```python
from build123d import *

# Parameters (mm, degrees)
PACK_PLINT_IZGARA_PANELI_1_START  = 18.5
SKETCH1_W                         = 580
SKETCH1_H                         = 80
PACK_PLINT_IZGARA_PANELI_1_DEPTH  = 1.5
PACK_PLINT_IZGARA_PANELI_2_START  = 17
SKETCH2_W                         = 20
SKETCH2_H                         = 60
PACK_PLINT_IZGARA_PANELI_2_DEPTH  = 4
PACK_PLINT_IZGARA_PANELI_3_START  = 17
SKETCH3_W                         = 20
SKETCH3_H                         = 60
PACK_PLINT_IZGARA_PANELI_3_DEPTH  = 4
PACK_PLINT_IZGARA_PANELI_4_START  = 17
SKETCH4_W                         = 20
SKETCH4_H                         = 60
PACK_PLINT_IZGARA_PANELI_4_DEPTH  = 4
PACK_PLINT_IZGARA_PANELI_5_START  = 17
SKETCH5_W                         = 20
SKETCH5_H                         = 60
PACK_PLINT_IZGARA_PANELI_5_DEPTH  = 4
PACK_PLINT_IZGARA_PANELI_6_START  = 17
SKETCH6_W                         = 20
SKETCH6_H                         = 60
PACK_PLINT_IZGARA_PANELI_6_DEPTH  = 4
PACK_PLINT_IZGARA_PANELI_7_START  = 17
SKETCH7_W                         = 20
SKETCH7_H                         = 60
PACK_PLINT_IZGARA_PANELI_7_DEPTH  = 4
PACK_PLINT_IZGARA_PANELI_8_START  = 17
SKETCH8_W                         = 20
SKETCH8_H                         = 60
PACK_PLINT_IZGARA_PANELI_8_DEPTH  = 4
PACK_PLINT_IZGARA_PANELI_9_START  = 17
SKETCH9_W                         = 20
SKETCH9_H                         = 60
PACK_PLINT_IZGARA_PANELI_9_DEPTH  = 4
PACK_PLINT_IZGARA_PANELI_10_START = 17
SKETCH10_W                        = 20
SKETCH10_H                        = 60
PACK_PLINT_IZGARA_PANELI_10_DEPTH = 4
PACK_PLINT_IZGARA_PANELI_11_START = 17
SKETCH11_W                        = 20
SKETCH11_H                        = 60
PACK_PLINT_IZGARA_PANELI_11_DEPTH = 4
PACK_PLINT_IZGARA_PANELI_12_START = 17
SKETCH12_W                        = 20
SKETCH12_H                        = 60
PACK_PLINT_IZGARA_PANELI_12_DEPTH = 4
PACK_PLINT_IZGARA_PANELI_13_START = 17
SKETCH13_W                        = 20
SKETCH13_H                        = 60
PACK_PLINT_IZGARA_PANELI_13_DEPTH = 4
PACK_PLINT_IZGARA_PANELI_14_START = 17
SKETCH14_W                        = 20
SKETCH14_H                        = 60
PACK_PLINT_IZGARA_PANELI_14_DEPTH = 4
PACK_PLINT_IZGARA_PANELI_15_START = 17
SKETCH15_W                        = 20
SKETCH15_H                        = 60
PACK_PLINT_IZGARA_PANELI_15_DEPTH = 4


with BuildPart() as part:
    # Sketch1 → PACK_plint_izgara_paneli_1 (new body)
    with BuildSketch(Plane.XY.offset(PACK_PLINT_IZGARA_PANELI_1_START)):
        with Locations((350, 70)):
            Rectangle(SKETCH1_W, SKETCH1_H)
    extrude(amount=PACK_PLINT_IZGARA_PANELI_1_DEPTH)

    # Sketch2 → PACK_plint_izgara_paneli_2 (cut)
    with BuildSketch(Plane.XY.offset(PACK_PLINT_IZGARA_PANELI_2_START)):
        with Locations((90, 70)):
            Rectangle(SKETCH2_W, SKETCH2_H)
    extrude(amount=PACK_PLINT_IZGARA_PANELI_2_DEPTH, mode=Mode.SUBTRACT)

    # Sketch3 → PACK_plint_izgara_paneli_3 (cut)
    with BuildSketch(Plane.XY.offset(PACK_PLINT_IZGARA_PANELI_3_START)):
        with Locations((130, 70)):
            Rectangle(SKETCH3_W, SKETCH3_H)
    extrude(amount=PACK_PLINT_IZGARA_PANELI_3_DEPTH, mode=Mode.SUBTRACT)

    # Sketch4 → PACK_plint_izgara_paneli_4 (cut)
    with BuildSketch(Plane.XY.offset(PACK_PLINT_IZGARA_PANELI_4_START)):
        with Locations((170, 70)):
            Rectangle(SKETCH4_W, SKETCH4_H)
    extrude(amount=PACK_PLINT_IZGARA_PANELI_4_DEPTH, mode=Mode.SUBTRACT)

    # Sketch5 → PACK_plint_izgara_paneli_5 (cut)
    with BuildSketch(Plane.XY.offset(PACK_PLINT_IZGARA_PANELI_5_START)):
        with Locations((210, 70)):
            Rectangle(SKETCH5_W, SKETCH5_H)
    extrude(amount=PACK_PLINT_IZGARA_PANELI_5_DEPTH, mode=Mode.SUBTRACT)

    # Sketch6 → PACK_plint_izgara_paneli_6 (cut)
    with BuildSketch(Plane.XY.offset(PACK_PLINT_IZGARA_PANELI_6_START)):
        with Locations((250, 70)):
            Rectangle(SKETCH6_W, SKETCH6_H)
    extrude(amount=PACK_PLINT_IZGARA_PANELI_6_DEPTH, mode=Mode.SUBTRACT)

    # Sketch7 → PACK_plint_izgara_paneli_7 (cut)
    with BuildSketch(Plane.XY.offset(PACK_PLINT_IZGARA_PANELI_7_START)):
        with Locations((290, 70)):
            Rectangle(SKETCH7_W, SKETCH7_H)
    extrude(amount=PACK_PLINT_IZGARA_PANELI_7_DEPTH, mode=Mode.SUBTRACT)

    # Sketch8 → PACK_plint_izgara_paneli_8 (cut)
    with BuildSketch(Plane.XY.offset(PACK_PLINT_IZGARA_PANELI_8_START)):
        with Locations((330, 70)):
            Rectangle(SKETCH8_W, SKETCH8_H)
    extrude(amount=PACK_PLINT_IZGARA_PANELI_8_DEPTH, mode=Mode.SUBTRACT)

    # Sketch9 → PACK_plint_izgara_paneli_9 (cut)
    with BuildSketch(Plane.XY.offset(PACK_PLINT_IZGARA_PANELI_9_START)):
        with Locations((370, 70)):
            Rectangle(SKETCH9_W, SKETCH9_H)
    extrude(amount=PACK_PLINT_IZGARA_PANELI_9_DEPTH, mode=Mode.SUBTRACT)

    # Sketch10 → PACK_plint_izgara_paneli_10 (cut)
    with BuildSketch(Plane.XY.offset(PACK_PLINT_IZGARA_PANELI_10_START)):
        with Locations((410, 70)):
            Rectangle(SKETCH10_W, SKETCH10_H)
    extrude(amount=PACK_PLINT_IZGARA_PANELI_10_DEPTH, mode=Mode.SUBTRACT)

    # Sketch11 → PACK_plint_izgara_paneli_11 (cut)
    with BuildSketch(Plane.XY.offset(PACK_PLINT_IZGARA_PANELI_11_START)):
        with Locations((450, 70)):
            Rectangle(SKETCH11_W, SKETCH11_H)
    extrude(amount=PACK_PLINT_IZGARA_PANELI_11_DEPTH, mode=Mode.SUBTRACT)

    # Sketch12 → PACK_plint_izgara_paneli_12 (cut)
    with BuildSketch(Plane.XY.offset(PACK_PLINT_IZGARA_PANELI_12_START)):
        with Locations((490, 70)):
            Rectangle(SKETCH12_W, SKETCH12_H)
    extrude(amount=PACK_PLINT_IZGARA_PANELI_12_DEPTH, mode=Mode.SUBTRACT)

    # Sketch13 → PACK_plint_izgara_paneli_13 (cut)
    with BuildSketch(Plane.XY.offset(PACK_PLINT_IZGARA_PANELI_13_START)):
        with Locations((530, 70)):
            Rectangle(SKETCH13_W, SKETCH13_H)
    extrude(amount=PACK_PLINT_IZGARA_PANELI_13_DEPTH, mode=Mode.SUBTRACT)

    # Sketch14 → PACK_plint_izgara_paneli_14 (cut)
    with BuildSketch(Plane.XY.offset(PACK_PLINT_IZGARA_PANELI_14_START)):
        with Locations((570, 70)):
            Rectangle(SKETCH14_W, SKETCH14_H)
    extrude(amount=PACK_PLINT_IZGARA_PANELI_14_DEPTH, mode=Mode.SUBTRACT)

    # Sketch15 → PACK_plint_izgara_paneli_15 (cut)
    with BuildSketch(Plane.XY.offset(PACK_PLINT_IZGARA_PANELI_15_START)):
        with Locations((610, 70)):
            Rectangle(SKETCH15_W, SKETCH15_H)
    extrude(amount=PACK_PLINT_IZGARA_PANELI_15_DEPTH, mode=Mode.SUBTRACT)


solid = part.part
```
The model under review builds one solid part; all positions refer to its coordinate system, in mm. Coordinates: 2 decimals unless noted, no trailing zeros. Write each loop counter-clockwise with the first axis right and the second up, starting at its lowest first coordinate (ties: lowest second). Pieces come first, ordered by that corner, then holes.
1) We need section B-B on y = 62.5. Count the separate pieces of the cut face and the enclosed holes in it, then the cut area to 3 significant figures.
2) We need section A-A on x = 286.5. State the section outline as (y, z) points.
3) To check wall thickness, follow probe 1 along Y at (x, z) = (454, 19.5). State the ranges of the line that lie inside material, in increasing order.
Answer list:
1. separate pieces: 15
1. enclosed holes: 0
1. area: 450 mm2
2. outline: (30, 18.5) - (40, 18.5) - (40, 20) - (30, 20) - close; (100, 18.5) - (110, 18.5) - (110, 20) - (100, 20) - close
3. probe 1: y = 30 to 40, 100 to 110
